Geometry check sheet. Reference: the model listing, model coordinates, mm. Face numbers are marked on the shaded views. A direction names the side the tool comes from. Round coordinates to 2 decimals unless told otherwise and drop trailing zeros. Write each loop counter-clockwise with the first axis right and the second up, starting at its lowest first coordinate (ties: lowest second). Pieces come first, ordered by that corner, then holes. Notation, with made-up numbers: (38.5, -7) - (65.5, -7) arc R32 ccw to (65.5, 25) - close; hole circle Ø3 at (86.5, 66.25). An arc over 180 degrees is marked (long way). Return JSON: item names as keys, results as strings.
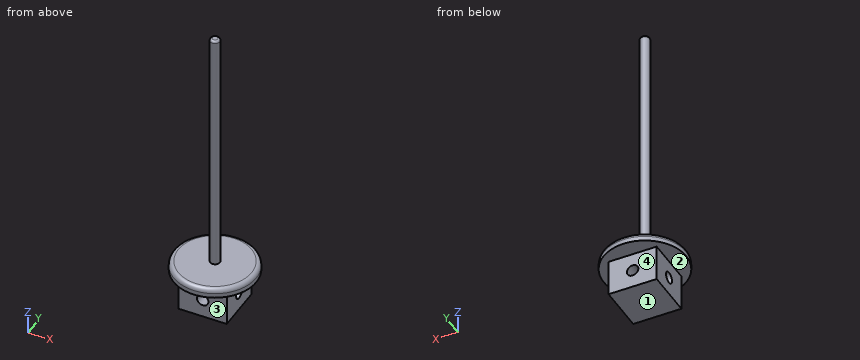
```python
from build123d import *

# Parameters (mm, degrees)
F0_R      = 18
F1_DEPTH  = 4
F2_W      = 21
F2_H      = 21
F3_DEPTH  = 16
F4_R      = 2.1
F5_DEPTH  = 20.001
F6_R      = 2
F7_R      = 2.1
F8_DEPTH  = 130
F9_R      = 1
F10_R     = 2.5
F11_DEPTH = 25
F12_R     = 2.5
F13_DEPTH = 25


with BuildPart() as f1:
    # F0 (on Top) → F1 (new body)
    with BuildSketch(Plane.XY):
        Circle(F0_R)
    extrude(amount=F1_DEPTH)

    # F2 (on Top) → F3 (join)
    with BuildSketch(Plane.XY):
        Rectangle(F2_W, F2_H)
    extrude(amount=-F3_DEPTH)

    # F4 (on face) → F5 (cut, through all)
    with BuildSketch(Plane.XY.offset(4)):
        Circle(F4_R)
    extrude(amount=-F5_DEPTH, mode=Mode.SUBTRACT)

    # F6
    f6_edges = [f1.edges().sort_by_distance(p)[0] for p in [
        (-18, 0, 4),
    ]]
    fillet(f6_edges, radius=F6_R)

    # F7 (on face) → F8 (join)
    with BuildSketch(Plane(origin=(0, 0, -16), x_dir=(1, 0, 0), z_dir=(0, 0, -1))):
        Circle(F7_R)
    extrude(amount=-F8_DEPTH)

    # F9
    f9_edges = [f1.edges().sort_by_distance(p)[0] for p in [
        (-2.1, 0, 114),
    ]]
    fillet(f9_edges, radius=F9_R)

    # F10 (on face) → F11 (cut)
    with BuildSketch(Plane.XZ.offset(10.5)):
        with Locations((0, -8)):
            Circle(F10_R)
    extrude(amount=-F11_DEPTH, mode=Mode.SUBTRACT)

    # F12 (on face) → F13 (cut)
    with BuildSketch(Plane(origin=(-10.5, 0, 0), x_dir=(0, -1, 0), z_dir=(-1, 0, 0))):
        with Locations((0, -8)):
            Circle(F12_R)
    extrude(amount=-F13_DEPTH, mode=Mode.SUBTRACT)


solid = f1.part
```
(1) Material ranges on line 1 along Z through (x, y) = (0, 7.25); line 2 along X through (y, z) = (3, -8), recorded low to high. Write a range as [from, to].
Response values:
{"line 1": "z = [-16, -10.5], [-5.5, 4]", "line 2": "x = [-10.5, -2.5], [2.5, 10.5]"}
(2) Access from +Z, -Z, +X, -X, +Y, -Y to the whole of each face (thin tool, end or side, straight path). Record for the marked faces 1, 2, 3 and 4.
Response values:
{"face 1": "-Z, +X, -X, +Y, -Y", "face 2": "-Z", "face 3": "-Z, +X, -X, -Y", "face 4": "-Z, +X, -X, +Y"}
(3) Gauge pin test, flat ends, axial feed: pin 1 (6.5 mm diameter, centred on y = 0, z = -8, fed in from +X); pin 2 (10 mm diameter, centred on y = 11.5, z = 92, fed in from -X); pin 3 (2 mm diameter, centred on x = 2.5, z = 91, fed in from +Y); pin 4 (6 mm diameter, centred on y = -4, z = 95.5, fed in from -X). Record the tip position at first contact, or that the pin passes through.
Response values:
{"pin 1": "stops at x = 10.5", "pin 2": "passes through", "pin 3": "stops at y = 1.47", "pin 4": "stops at x = -1.85"}
(4) Section check A-A, the plane z = -8. Enter the section's corners in (x, y), plus the area to 3 significant figures.
Response values:
{"outline": "(-10.5, -10.5) - (-2.5, -10.5) - (-2.5, -2.5) - (-10.5, -2.5) - close; (-10.5, 2.5) - (-2.5, 2.5) - (-2.5, 10.5) - (-10.5, 10.5) - close; (2.5, -10.5) - (10.5, -10.5) - (10.5, -2.5) - (2.5, -2.5) - close; (2.5, 2.5) - (10.5, 2.5) - (10.5, 10.5) - (2.5, 10.5) - close", "area": "256 mm^2"}
(5) Section check B-B, the plane z = 62.5. Enter the section's corners in (x, y).
Response values:
{"outline": "circle Ø4.2 at (0, 0)"}
